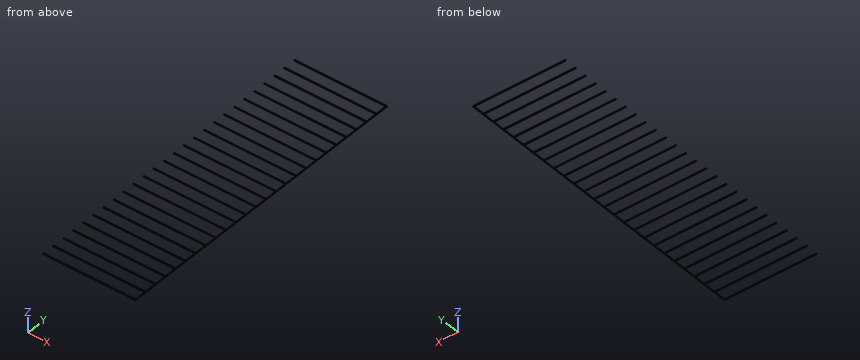
```python
from build123d import *

# Parameters (mm, degrees)
SKETCH004_R            = 0.25
PAD001_DEPTH           = 250
SKETCH003_R            = 0.25
PAD002_DEPTH           = 74
LINEARPATTERN002_COUNT = 26
LINEARPATTERN002_PITCH = 10


with BuildPart() as part:
    # Sketch004 → Pad001 (new body)
    with BuildSketch(Plane(origin=(37, 0, 0), x_dir=(1, 0, 0), z_dir=(0, -1, 0))):
        Circle(SKETCH004_R)
    extrude(amount=-PAD001_DEPTH)

    # Sketch003 → Pad002 (join)
    with BuildSketch(Plane.YZ.offset(37)):
        Circle(SKETCH003_R)
    pad002 = extrude(amount=-PAD002_DEPTH)

    # LinearPattern002: Pad002 ×26
    with Locations(*[(0, i * LINEARPATTERN002_PITCH, 0) for i in range(1, LINEARPATTERN002_COUNT)]):
        add(pad002)


with BuildPart() as part_1:
    # Body001 placement: moved
    add(part.part.moved(Location((0, 5, 2))))


solid = part_1.part
```
Part model, mm, in its own coordinate system. Give positions to 0.01 mm unless a question says otherwise; leave off trailing zeros. Write each loop counter-clockwise with the first axis right and the second up, starting at its lowest first coordinate (ties: lowest second). Pieces come first, ordered by that corner, then holes. Notation, with made-up numbers: (6, -20.5) -> (25, -20.5) arc R10 cw to (25, -12.5) -> close; hole circle Ø2 at (47, -7). An arc over 180 degrees is marked (long way). Put each result on its own line as item: value. Start each with the question number.
Item 1: Cut at A-A (x = -19.5). State how many separate pieces and enclosed holes the cut face has, then the cut area to 3 significant figures.
Item 2: Cut at B-B (y = 111). List the corners of the cut face in (x, z), then the cut area to 3 significant figures.
Item 3: Wall check: L1, parallel to X at y = 157.5, z = 1.9; L2, parallel to X at y = 215, z = 2.05. Give the ranges that are in metal, low to high. Write a range as [from, to].
Answer list:
1. separate pieces: 26
1. enclosed holes: 0
1. area: 5.11 mm2
2. outline: circle Ø0.5 at (37, 2)
2. area: 0.196 mm2
3. L1: x = [36.77, 37.23]
3. L2: x = [-37, 37.24]
